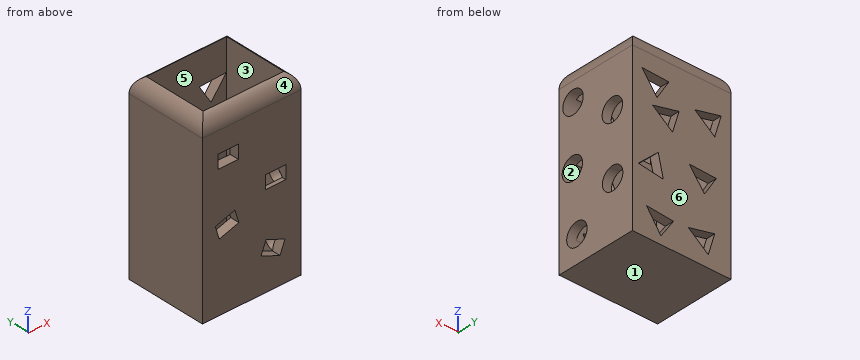
from build123d import *

# Parameters (mm, degrees)
F0_W        = 27.615731582
F0_H        = 22.7759163827
F1_DEPTH    = 51.308
F2_T        = -2.54
F3_T1_DEPTH = 53.015731582
F3_T3_DEPTH = 48.1759163827
F4_W        = 5.7445205748
F4_H        = 3.7603080273
F5_DEPTH    = 4.826
F7_D        = 6.35
F7_DEPTH    = 12.7
F7_TIP      = 1.9077324654
F9_DEPTH    = 8.382


# Not quite as in the source:
# - a fillet or chamfer that OpenCascade refuses, or shapes differently, is made with other operations: its cross-section is extruded or revolved along the edge and cut away or added


with BuildPart() as f1:
    # F0 (on Top) → F1 (new body)
    with BuildSketch(Plane.XY):
        with Locations((-13.807865791, 11.3879581913)):
            Rectangle(F0_W, F0_H)
    extrude(amount=F1_DEPTH)

    # F2
    f2_openings = [f1.faces().sort_by_distance(p)[0] for p in [
        (-13.807866, 11.387958, 51.308),
    ]]
    offset(amount=F2_T, openings=f2_openings)

    # F3: fillet of radius 5.08 on 4 edges, made by hand

    # F3_s2 → F3_t1 (cut)
    with BuildSketch(Plane.YZ.offset(-40.315731582)):
        with BuildLine():
            ThreePointArc((0, 46.228), (1.4878975516, 49.8201024484), (5.08, 51.308))
            Line((5.08, 51.308), (0, 51.308))
            Line((0, 51.308), (0, 46.228))
        make_face()
        with BuildLine():
            ThreePointArc((22.7759163827, 46.228), (21.2880188311, 49.8201024484), (17.6959163827, 51.308))
            Line((17.6959163827, 51.308), (22.7759163827, 51.308))
            Line((22.7759163827, 51.308), (22.7759163827, 46.228))
        make_face()
    extrude(amount=F3_T1_DEPTH, mode=Mode.SUBTRACT)

    # F3_s4 → F3_t3 (cut)
    with BuildSketch(Plane.XZ.offset(-35.4759163827)):
        with BuildLine():
            ThreePointArc((-27.615731582, 46.228), (-26.1278340305, 49.8201024484), (-22.535731582, 51.308))
            Line((-22.535731582, 51.308), (-27.615731582, 51.308))
            Line((-27.615731582, 51.308), (-27.615731582, 46.228))
        make_face()
        with BuildLine():
            ThreePointArc((0, 46.228), (-1.4878975516, 49.8201024484), (-5.08, 51.308))
            Line((-5.08, 51.308), (0, 51.308))
            Line((0, 51.308), (0, 46.228))
        make_face()
    extrude(amount=F3_T3_DEPTH, mode=Mode.SUBTRACT)

    # F4 (on face) → F5 (cut)
    with BuildSketch(Plane.XZ):
        with Locations((-20.4156730324, 38.4546555579)):
            Rectangle(F4_W, F4_H)
        with Locations((-7.0931273513, 27.5189299136)):
            Rectangle(F4_W, F4_H)
        Polygon((-18.5130548821, 24.3505493797), (-23.9980506161, 22.6434060253), (-22.880570963, 19.0529804677), (-17.395575229, 20.7601238221), align=None)
        Polygon((-4.4602522607, 10.9747632246), (-9.781830883, 13.1381673943), (-11.1979744862, 9.6547131094), (-5.8763958639, 7.4913089397), align=None)
    extrude(amount=-F5_DEPTH, mode=Mode.SUBTRACT)

    # F7
    with Locations(Plane.YZ):
        with Locations((4.3385280296, 40.9476608038), (16.5516659617, 33.1388860941), (4.1396417655, 24.540392682), (16.6495069861, 16.0039383918), (5.5445204489, 7.5149172917)):
            Hole(F7_D / 2, depth=F7_DEPTH)
            with Locations((0, 0, -(F7_DEPTH + F7_TIP / 2))):  # 118° drill point
                Cone(0, F7_D / 2, F7_TIP, mode=Mode.SUBTRACT)

    # F8 (on face) → F9 (cut)
    with BuildSketch(Plane(origin=(0, 22.7759163827, 0), x_dir=(-1, 0, 0), z_dir=(0, 1, 0))):
        Polygon((13.0775338039, 35.4098752141), (5.6731416844, 33.7212570012), (11.2572079524, 29.4185951352), align=None)
        Polygon((23.5141057819, 23.2905662243), (15.9249656523, 23.5758839796), (20.2051486408, 17.9745690622), align=None)
        Polygon((7.2458156385, 22.6723130022), (1.6777330699, 17.5077306728), (8.6650072474, 16.573549327), align=None)
        Polygon((23.0783666484, 9.331129957), (15.6739745289, 7.6425117441), (21.258040797, 3.3398498781), align=None)
        Polygon((11.5244448229, 7.3593156172), (3.9536968494, 7.9595066297), (7.997608447, 2.1852989602), align=None)
        Polygon((24.8908895689, 39.4682685534), (17.4864974494, 37.7796503405), (23.0705637174, 33.4769884745), align=None)
        Polygon((10.2386324033, 41.4962964688), (2.6494922737, 41.7816142241), (6.9296752622, 36.1802993067), align=None)
    extrude(amount=-F9_DEPTH, mode=Mode.SUBTRACT)


solid = f1.part
The model under review builds one solid part; all positions refer to its coordinate system, in mm. Face numbers are marked on the shaded views. A direction names the side the tool comes from. Give positions to 0.01 mm unless a question says otherwise; leave off trailing zeros. Order: outer loops, then holes, each group sorted by start corner. A loop starts at its lowest first (then second) coordinate and runs counter-clockwise, first axis right, second up. Notation, with made-up numbers: M 83,3 L 126,3 A32 ccw 126,40 Z; hole C -25,-25 d9. An arc over 180 degrees is marked long. Answer in a Markdown table with one row per item. Add a question column.
1. Add section C-C on y = 5. State the section outline as (x, z) points, plus the area to 3 significant figures.
2. Machinability: for the marked faces 5 and 6, which of the approach directions +Z, -Z, +X, -X, +Y, -Y give a long, thin tool a straight path to every point of the face, cutting with its end or side? Answer none if there is none.
3. Mouldability with a two-part tool opening along Z and no side actions: class the marked faces 1, 2, 3 and 4 as released by +Z, released by -Z, zero draft, split by the parting line, or undercut.
4. Add section D-D on x = -19.5. State the section outline as (y, z) points.
5. Add section A-A on y = 15.75. State the section outline as (x, z) points.
6. To check wall thickness, follow line 1 along Y through (x, z) = (-21, 31); line 2 along X through (y, z) = (18.5, 36); line 3 along Y through (x, z) = (-6.5, 21). State the ranges of each line that lie inside material, in increasing order.
7. Add section B-B on z = 30.5. State the section outline as (x, y) points.
8. For pin 1 Ø10 at (y, z) = (4.34, 40.95) entering from +X; pin 2 Ø0.6 at (x, y) = (-7, 1) entering from +Z, all flat-tipped, find the tip position at first contact; note any pin that passes through.
The answers:
| question | item | result |
|---|---|---|
| 1 | outline | M -27.62,0 L 0,0 L 0,4.39 L -2.54,4.39 L -2.54,2.54 L -25.08,2.54 L -25.08,50.63 A5.08 ccw -27.62,46.23 Z; M -2.54,10.64 L 0,10.64 L 0,21.48 L -2.54,21.48 Z; M -2.54,27.6 L 0,27.6 L 0,37.84 L -2.54,37.84 Z; M -2.54,44.05 L 0,44.05 L 0,46.23 A5.08 ccw -2.54,50.63 Z |
| 1 | area | 261 mm2 |
| 2 | face 5 | +Z |
| 2 | face 6 | +Z, -Z, +X, -X, +Y |
| 3 | face 1 | released by -Z |
| 3 | face 2 | undercut |
| 3 | face 3 | zero draft |
| 3 | face 4 | released by +Z |
| 4 | outline | M 0,0 L 22.78,0 L 22.78,4.69 L 20.24,4.69 L 20.24,2.54 L 2.54,2.54 L 2.54,20.11 L 0,20.11 Z; M 0,24.04 L 2.54,24.04 L 2.54,36.57 L 0,36.57 Z; M 0,40.33 L 2.54,40.33 L 2.54,50.63 A5.08 ccw 0,46.23 Z; M 20.24,8.52 L 22.78,8.52 L 22.78,18.9 L 20.24,18.9 Z; M 20.24,23.44 L 22.78,23.44 L 22.78,36.23 L 20.24,36.23 Z; M 20.24,38.24 L 22.78,38.24 L 22.78,46.23 A5.08 ccw 20.24,50.63 Z |
| 5 | outline | M -27.62,0 L 0,0 L 0,12.96 L -2.54,12.96 L -2.54,2.54 L -7.75,2.54 L -8,2.19 L -8.24,2.54 L -25.08,2.54 L -25.08,50.63 A5.08 ccw -27.62,46.23 Z; M -2.54,19.05 L 0,19.05 L 0,30.07 L -2.54,30.07 Z; M -2.54,36.21 L 0,36.21 L 0,46.23 A5.08 ccw -2.54,50.63 Z |
| 6 | line 1 | 0 to 2.54, 20.24 to 22.78 |
| 6 | line 2 | -27.62 to -25.08, -2.54 to 0 |
| 6 | line 3 | 0 to 2.54 |
| 7 | outline | M -27.62,0 L 0,0 L 0,14.79 L -2.54,14.79 L -2.54,2.54 L -25.08,2.54 L -25.08,20.24 L -11.59,20.24 L -11.59,22.78 L -27.62,22.78 Z; M -9.85,20.24 L -2.54,20.24 L -2.54,18.32 L 0,18.32 L 0,22.78 L -9.85,22.78 Z |
| 8 | pin 1 | x = 0 |
| 8 | pin 2 | z = 49.62 |
